Drawing for the job (mm, zero at the part's lowest x, y, z). Coordinates: 2 decimals unless noted, no trailing zeros. Loops run counter-clockwise (first coordinate to the right, second up) from the corner with the lowest first, then second, coordinate; pieces in that order, holes last. Notation, with made-up numbers: (87, -7.75) -> (145, -7.75) arc R6 ccw to (145, -1.75) -> close; hole circle Ø8 at (-7.75, -15.5). An arc over 180 degrees is marked (long way). Write each question's results on one line, items separated by ' | '.
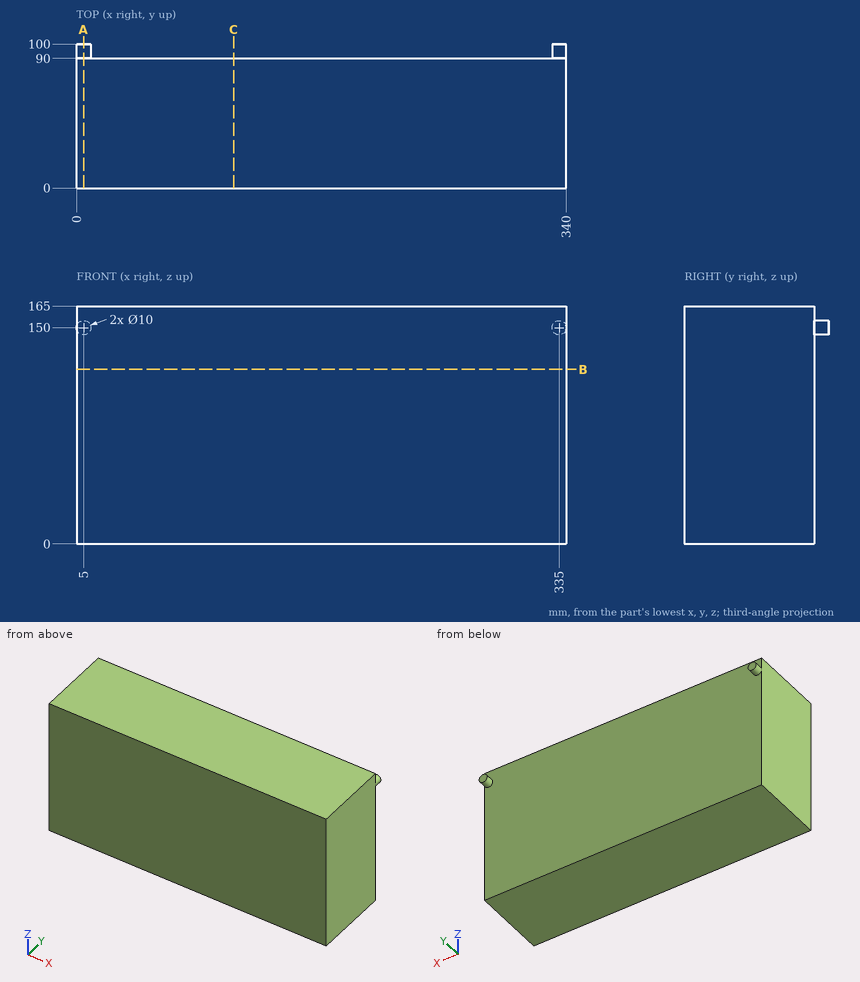
1) Slice it at A-A (x = 5). Write the cut outline in (y, z).
Outcome:
outline: (0, 0) -> (90, 0) -> (90, 145) -> (100, 145) -> (100, 155) -> (90, 155) -> (90, 165) -> (0, 165) -> close
2) Drill centre line: L1, parallel to Y at x = 250.5, z = 88. Where is it in solid material? Low to high. Write a range as from..to.
Outcome:
L1: y = 0..90
3) Slice it at C-C (x = 109). Write the cut outline in (y, z), then the cut area to 4 significant figures.
Outcome:
outline: (0, 0) -> (90, 0) -> (90, 165) -> (0, 165) -> close | area: 14,850 mm^2
4) Slice it at B-B (z = 121). Write the cut outline in (x, y).
Outcome:
outline: (0, 0) -> (340, 0) -> (340, 90) -> (0, 90) -> close
5) Pin check, flat tips, straight feed: pin 1 (3 mm diameter, centred on x = 277, z = 80.5, fed in from -Y); pin 2 (10 mm diameter, centred on x = 300.5, z = 148.5, fed in from +Y). Stop position of each tip, or through.
Outcome:
pin 1: stops at y = 0 | pin 2: stops at y = 90
